Work out the finished part from the listing and answer in its coordinate system (mm). Face numbers are marked on the shaded views. A direction names the side the tool comes from. Coordinates: 2 decimals unless noted, no trailing zeros. Write each loop counter-clockwise with the first axis right and the second up, starting at its lowest first coordinate (ties: lowest second). Pieces come first, ordered by that corner, then holes. Notation, with made-up numbers: (-16, 63) - (-2, 63) arc R15 cw to (-2, 83) - close; hole circle Ø7 at (24.5, 71). An arc over 180 degrees is marked (long way). One line per item, written item: value.
```python
from build123d import *
from build123d.topology import SkipClean

# Parameters (mm, degrees)
SKETCH1_R               = 38.1
SKETCH1_R_2             = 31.75
BOSS_EXTRUDE1_DEPTH     = 63.5
SKETCH2_R               = 50.8
BOSS_EXTRUDE2_DEPTH     = 10.16
CUT_EXTRUDE2_DEPTH      = 53.34
CUT_EXTRUDE2_DEPTH_BACK = 96.882897328
SKETCH3_R               = 31.75
BOSS_EXTRUDE3_START     = 10.16
SKETCH4_R               = 38.1
SKETCH4_R_2             = 31.75
BOSS_EXTRUDE3_DEPTH     = 10.16


with BuildPart() as part:
    # Sketch1 → Boss-Extrude1 (new body)
    with BuildSketch(Plane.XY):
        Circle(SKETCH1_R)
        Circle(SKETCH1_R_2, mode=Mode.SUBTRACT)
    extrude(amount=BOSS_EXTRUDE1_DEPTH)

    # Sketch2 → Boss-Extrude2 (add)
    with BuildSketch(Plane(origin=(0, 0, 0), x_dir=(-1, 0, 0), z_dir=(0, 0, -1))):
        Circle(SKETCH2_R)
    extrude(amount=BOSS_EXTRUDE2_DEPTH)

    # Sketch3 → Cut-Extrude2 (cut, two sides: drawn at the far end of the back side and taken through both)
    with SkipClean():  # the faces are left unmerged after this step: merging them gives an invalid solid
        with BuildSketch(Plane(origin=(0, 0, 0), x_dir=(-1, 0, 0), z_dir=(0, 0, -1)).offset(-CUT_EXTRUDE2_DEPTH_BACK)):
            Circle(SKETCH3_R)
        extrude(amount=CUT_EXTRUDE2_DEPTH + CUT_EXTRUDE2_DEPTH_BACK, mode=Mode.SUBTRACT)
    add(part.part.scale(1), mode=Mode.REPLACE)  # the faces are merged on a copy

    # Sketch4 → Boss-Extrude3 (add)
    with BuildSketch(Plane(origin=(0, 0, -10.16), x_dir=(-1, 0, 0), z_dir=(0, 0, -1)).offset(BOSS_EXTRUDE3_START)):
        Circle(SKETCH4_R)
        Circle(SKETCH4_R_2, mode=Mode.SUBTRACT)
    extrude(amount=-BOSS_EXTRUDE3_DEPTH)


solid = part.part
```
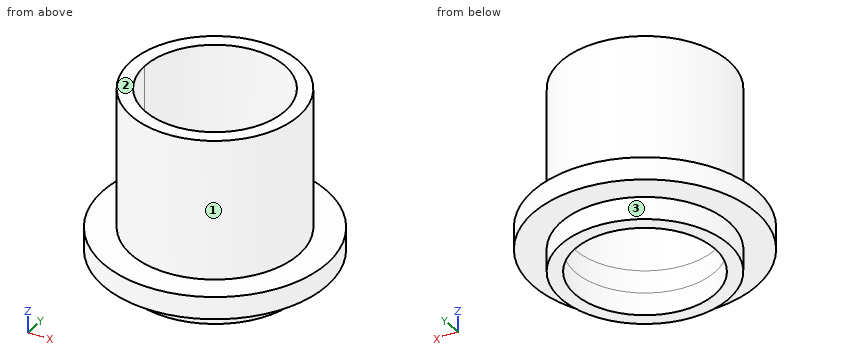
Item 1: Given pin 1 (12 mm diameter, centred on x = 32.5, z = 42, fed in from -Y); pin 2 (2 mm diameter, centred on x = 19, z = 50, fed in from +Y); pin 3 (5 mm diameter, centred on y = 11, z = 11.5, fed in from -X), each flat-ended and moving along its own axis, determine where each tip first touches the part or whether it passes through.
Evaluation:
pin 1: stops at y = -27.37
pin 2: stops at y = 33.58
pin 3: stops at x = -37.14
Item 2: Consider probe 1 along Y at (x, z) = (0, -8); probe 2 along Y at (x, z) = (0, -13); probe 3 along X at (y, z) = (-11, 38.5). Determine where each line is inside the solid, lowest interval first.
Evaluation:
probe 1: y = -50.8 to -31.75, 31.75 to 50.8
probe 2: y = -38.1 to -31.75, 31.75 to 38.1
probe 3: x = -36.48 to -29.78, 29.78 to 36.48
Item 3: Section B-B, the plane y = -4.5 is taken. Determine the outline of the cut face in (x, z).
Evaluation:
outline: (-50.6, -10.16) - (-37.83, -10.16) - (-37.83, -20.32) - (-31.43, -20.32) - (-31.43, 63.5) - (-37.83, 63.5) - (-37.83, 0) - (-50.6, 0) - close; (31.43, -20.32) - (37.83, -20.32) - (37.83, -10.16) - (50.6, -10.16) - (50.6, 0) - (37.83, 0) - (37.83, 63.5) - (31.43, 63.5) - close
Item 4: Which of the six approach directions +Z, -Z, +X, -X, +Y, -Y give full straight-line access (tool end or side, diameter ignored) to the marked faces 1, 2 and 3?
Evaluation:
face 1: +Z
face 2: +Z, +X, -X, +Y, -Y
face 3: -Z
Item 5: Section D-D, the plane y = 35 is taken. Determine the outline of the cut face in (x, z).
Evaluation:
outline: (-36.82, -10.16) - (-15.05, -10.16) - (-15.05, -20.32) - (15.05, -20.32) - (15.05, -10.16) - (36.82, -10.16) - (36.82, 0) - (15.05, 0) - (15.05, 63.5) - (-15.05, 63.5) - (-15.05, 0) - (-36.82, 0) - close
Item 6: Section A-A, the plane x = 0 is taken. Determine the outline of the cut face in (y, z).
Evaluation:
outline: (-50.8, -10.16) - (-38.1, -10.16) - (-38.1, -20.32) - (-31.75, -20.32) - (-31.75, 63.5) - (-38.1, 63.5) - (-38.1, 0) - (-50.8, 0) - close; (31.75, -20.32) - (38.1, -20.32) - (38.1, -10.16) - (50.8, -10.16) - (50.8, 0) - (38.1, 0) - (38.1, 63.5) - (31.75, 63.5) - close
Item 7: Section C-C, the plane z = -7 is taken. Determine the outline of the cut face in (x, y), then the cut area to 3 significant figures.
Evaluation:
outline: circle Ø101.6 at (0, 0); hole circle Ø63.5 at (0, 0)
area: 4,940 mm2
